from build123d import *


with BuildPart() as part:
    # Body Sketch → Body Revolve (revolve)
    with BuildSketch(Plane(origin=(0, 0, 0), x_dir=(1, 0, 0), z_dir=(0, 1, 0)), mode=Mode.PRIVATE) as body_revolve_sk:
        Polygon((2.65, -14.5), (3.1, -14.5), (3.1, -12), (5.225, -12), (5.225, -11), (3.1, -11), (3.1, -5.7), (1.625, -5.3), (1.625, -3.9), (2.5, -3.9), (2.5, -3.15), (1.25, -3.15), (1, -0.75), (0.775, -0.75), (0.775, 0), (0.25, 0), (0.25, -5.704207714), (2.65, -6.355055172), align=None)
    revolve(body_revolve_sk.sketch.rotate(Axis((0, 0, 0), (0, 0, 1)), 180), axis=Axis((0, 0, 0), (0, 0, 1)))


solid = part.part
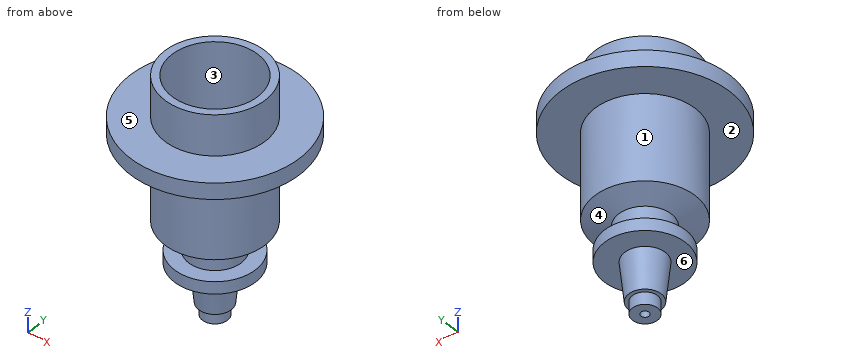
Build history of the part. All positions in model axes, mm. Face numbers are marked on the shaded views. A direction names the side the tool comes from. Give positions to 0.01 mm unless a question says otherwise; leave off trailing zeros. Loops run counter-clockwise (first coordinate to the right, second up) from the corner with the lowest first, then second, coordinate; pieces in that order, holes last. Notation, with made-up numbers: (-13, -40) -> (1, -40) arc R12 cw to (1, -18) -> close; hole circle Ø6 at (73, -11). An arc over 180 degrees is marked (long way). Answer in a Markdown table with one row per item.
Item 1: Slice it at D-D on y = 4.25. Write the cut outline in (x, z).
Findings below:
| item | result |
|---|---|
| outline | (-3.04, 11) -> (3.04, 11) -> (3.04, 12) -> (-3.04, 12) -> close |
Item 2: Flat gauge pins, fed straight in: P1, Ø3, axis at y = 1.5, z = 3, coming from the +X side; P2, Ø6, axis at x = 2.5, y = -4, coming from the -Z side; P3, Ø3, axis at x = 2, y = 4, coming from the -Z side. Where does each tip first touch, or does it go through?
Findings below:
| item | result |
|---|---|
| P1 | stops at x = 2.5 |
| P2 | stops at z = 3.15 |
| P3 | stops at z = 5.67 |
Item 3: Mould opens along Y. For the marked faces 1, 2 and 3 say: pulls with the +Y half, pulls with the -Y half, needs draft (parallel to the pull), parting line crosses it, or undercut.
Findings below:
| item | result |
|---|---|
| face 1 | parting line crosses it |
| face 2 | needs draft |
| face 3 | undercut |
Item 4: Probe line 1 along Y through (x, z) = (0.75, 7.75); line 2 along Y through (x, z) = (0, 2.2); line 3 along Z through (x, y) = (2, -1.25). List the from-to ranges inside material, lowest first. Write a range as [from, to].
Findings below:
| item | result |
|---|---|
| line 1 | y = [-3.01, -2.54], [2.54, 3.01] |
| line 2 | y = [-1.15, -0.25], [0.25, 1.15] |
| line 3 | z = [3.15, 3.9], [5.5, 6.28] |
Item 5: Slice it at B-B on y = -3.5. Write the cut outline in (x, z).
Findings below:
| item | result |
|---|---|
| outline | (-3.88, 11) -> (3.88, 11) -> (3.88, 12) -> (-3.88, 12) -> close |
Item 6: Slice it at C-C on z = 2.5. Write the cut outline in (x, y).
Findings below:
| item | result |
|---|---|
| outline | circle Ø2.36 at (0, 0); hole circle Ø0.5 at (0, 0) |
Item 7: Slice it at A-A on z = 9.5. Write the cut outline in (x, y).
Findings below:
| item | result |
|---|---|
| outline | circle Ø6.2 at (0, 0); hole circle Ø5.3 at (0, 0) |
Item 8: Tool access for the marked faces 4, 5 and 6: list every direction of +Z, -Z, +X, -X, +Y, -Y with a clear straight run to the whole face (end or side of a thin tool).
Findings below:
| item | result |
|---|---|
| face 4 | none |
| face 5 | +Z |
| face 6 | -Z |
